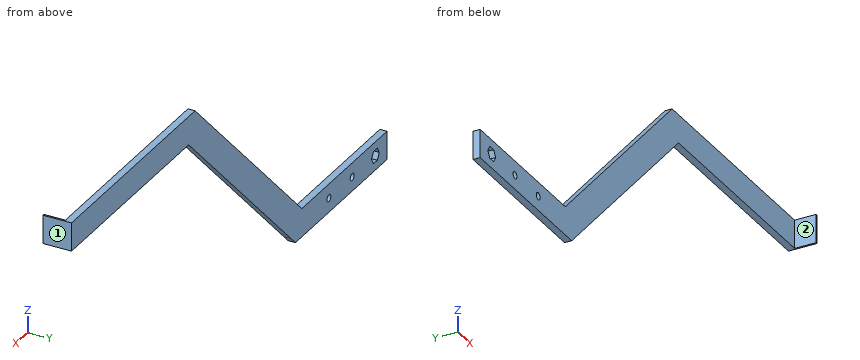
Autodesk Inventor part; units mm, degrees
ref_plane "YZ Plane" through (0, 0, 0) normal (1, 0, 0) x (0, 1, 0)
ref_plane "XZ Plane" through (0, 0, 0) normal (0, 1, 0) x (-1, 0, 0)
ref_plane "XY Plane" through (0, 0, 0) normal (0, 0, 1) x (1, 0, 0)
sketch "Sketch1" plane through (0, 0, 0) normal (0, 1, 0) x (-1, 0, 0)
  line L0 (0, 0) -> (-133.35, 0)
  line L1 (-133.35, 0) -> (-133.35, 25.4)
  line L2 (-133.35, 25.4) -> (0, 25.4)
  line L3 (0, 25.4) -> (0, 0)
  line L4 (-133.35, 25.4) -> (-143.871, 0)
  line L5 (-133.35, 25.4) -> (-105.8572, 25.4) construction
  line L6 (-133.35, 25.4) -> (-151.3105, 7.4395)
  line L7 (-133.35, 25.4) -> (-107.95, 25.4) construction
  line L8 (-151.3105, 7.4395) -> (-143.871, 0)
  line L9 (-133.35, 25.4) -> (-151.3105, 7.4395)
  line L10 (-151.3105, 7.4395) -> (-318.9899, 175.1188)
  line L11 (-318.9899, 175.1188) -> (-301.0293, 193.0793)
  line L12 (-301.0293, 193.0793) -> (-133.35, 25.4)
  circle A0 centre (-12.7, 12.7) radius 6.35
  line L13 (-318.9899, 175.1188) -> (-509.4899, 175.1188)
  line L14 (-509.4899, 175.1188) -> (-509.4899, 200.5188)
  line L15 (-509.4899, 200.5188) -> (-318.9899, 200.5188)
  line L16 (-318.9899, 200.5188) -> (-318.9899, 175.1188)
  line L17 (-318.9899, 175.1188) -> (-308.4688, 200.5188)
  line L18 (-308.4688, 200.5188) -> (-318.9899, 200.5188)
  line L19 (-308.4688, 200.5188) -> (-301.0293, 193.0793)
  line L20 (-133.35, 0) -> (-143.871, 0)
  dimension "d0" = 133.35
  dimension "d1" = 25.4
  dimension "d2" = 112.5
  dimension "d3" = 25.4
  dimension "d4" = 135
  dimension "d5" = 237.1344
  dimension "d6" = 12.7
  dimension "d7" = 190.5
  dimension "d8" = 25.4
extrude "Extrusion1" add sketch "Sketch1" along normal blind 6.35
sketch "Sketch2" plane through (509.4899, 0, 200.5188) normal (1, 0, 0) x (0, 0, -1)
  line L0 (0, 6.35) -> (25.4, 6.35)
  line L1 (25.4, 6.35) -> (25.4, -19.05)
  line L2 (25.4, -19.05) -> (0, -19.05)
  line L3 (0, -19.05) -> (0, 6.35)
  point P0 (200.5188, 0)
  dimension "d11" = 25.4
  dimension "d12" = 25.4
extrude "Extrusion2" add sketch "Sketch2" along normal blind 1.5875
sketch "Sketch3" plane through (0, 0, 0) normal (-1, 0, 0) x (0, 0, 1)
  line L0 (0, 0) -> (25.4, 0)
  line L1 (25.4, 0) -> (25.4, 6.35)
  line L2 (0, 6.35) -> (25.4, 6.35)
  line L3 (0, 0) -> (0, 6.35)
extrude "Extrusion3" add sketch "Sketch3" along normal blind 44.45
sketch "Sketch6" plane through (0, 6.35, 0) normal (0, 1, 0) x (1, 0, 0)
  circle A0 centre (12.7, -12.7) radius 6.35
  line L0 (318.9899, -175.1188) -> (511.0774, -175.1188)
  line L1 (12.7, -12.7) -> (12.7, -6.35)
  line L2 (16.3662, -6.35) -> (20.0323, -12.7)
  line L3 (20.0323, -12.7) -> (16.3662, -19.05)
  line L4 (16.3662, -19.05) -> (9.0338, -19.05)
  line L5 (9.0338, -19.05) -> (5.3677, -12.7)
  line L6 (5.3677, -12.7) -> (9.0338, -6.35)
  line L7 (9.0338, -6.35) -> (16.3662, -6.35)
  point P0 (0, 0)
extrude "Extrusion5" cut sketch "Sketch6" against normal blind 6.35 contours A0 L2 L3 | A0 L7 L2 | L3 L4 A0 | A0 L6 L7 | L4 L5 A0 | A0 L5 L6
sketch "Sketch8" plane through (0, 6.35, 0) normal (0, 1, 0) x (1, 0, 0)
  line L0 (143.871, 0) -> (-44.45, 0)
  line L1 (-44.45, -25.4) -> (-44.45, 0)
  line L2 (318.9899, -175.1188) -> (511.0774, -175.1188)
  line L3 (-44.45, -12.7) -> (12.7, -12.7)
  line L4 (12.7, -12.7) -> (12.7, 0)
  line L5 (12.7, -12.7) -> (-25.4, -12.7)
  line L6 (-25.4, -12.7) -> (50.8, -12.7)
  circle A0 centre (-25.4, -12.7) radius 3.175
  circle A1 centre (50.8, -12.7) radius 3.175
  point P0 (0, 0)
  dimension "d29" = 57.15
  dimension "d30" = 38.1
  dimension "d31" = 76.2
  dimension "d32" = 0
  dimension "d33" = 6.35
  dimension "d34" = 6.35
extrude "Extrusion7" cut sketch "Sketch8" against normal blind 25.4 contours A1 | A0 L3 | L3 A0
sketch "Sketch9" plane through (0, 6.35, 0) normal (0, 1, 0) x (1, 0, 0)
  circle A0 centre (50.8, -12.7) radius 3.175
  circle A1 centre (-25.4, -12.7) radius 3.175
  line L0 (-44.45, 0) -> (0, 0)
  line L1 (0, 0) -> (0, -25.4)
  line L2 (0, -25.4) -> (-44.45, -25.4)
  line L3 (-44.45, -25.4) -> (-44.45, 0)
  line L4 (0, -12.7) -> (12.7, -12.7)
  line L5 (12.7, -12.7) -> (50.8, -12.7)
  line L6 (50.8, -12.7) -> (88.9, -12.7)
  line L7 (50.8, -12.7) -> (88.9, -12.7) construction
  circle A2 centre (88.9, -12.7) radius 3.175
  dimension "d37" = 44.45
  dimension "d38" = 25.4
  dimension "d39" = 38.1
  dimension "d40" = 0
  dimension "d41" = 6.35
extrude "Extrusion8" cut sketch "Sketch9" against normal blind 25.4 contours L1 L2 L3 L0 | A2
sketch "Sketch10" plane through (0, 6.35, 0) normal (-1, 0, 0) x (0, 0, 1)
  line L0 (25.4, -6.35) -> (0, -6.35)
  line L1 (25.4, 0) -> (25.4, -6.35)
  line L2 (0, 0) -> (25.4, 0)
  line L3 (0, -6.35) -> (0, 0)
extrude "Extrusion9" add sketch "Sketch10" along normal blind 6.35
sketch "Sketch11" plane through (0, 6.35, 0) normal (0, 1, 0) x (1, 0, 0)
  line L0 (-6.35, -25.4) -> (-6.35, 0)
  line L1 (5.3677, -12.7) -> (9.0338, -6.35)
  line L2 (9.0338, -6.35) -> (16.3662, -6.35)
  line L3 (16.3662, -6.35) -> (20.0323, -12.7)
  line L4 (20.0323, -12.7) -> (16.3662, -19.05)
  line L5 (16.3662, -19.05) -> (9.0338, -19.05)
  line L6 (9.0338, -19.05) -> (5.3677, -12.7)
  line L7 (-6.35, -12.7) -> (12.7, -12.7)
  line L8 (12.7, -12.7) -> (6.35, -12.7)
  line L9 (12.7, -12.7) -> (19.05, -12.7) construction
  line L10 (6.35, -12.7) -> (9.525, -7.2007)
  line L11 (9.525, -7.2007) -> (15.875, -7.2007)
  line L12 (15.875, -7.2007) -> (19.05, -12.7)
  line L13 (19.05, -12.7) -> (15.875, -18.1993)
  line L14 (15.875, -18.1993) -> (9.525, -18.1993)
  line L15 (9.525, -18.1993) -> (6.35, -12.7)
  point P0 (0, 0)
  dimension "d46" = 6.35
  dimension "d47" = 180
extrude "Extrusion10" add sketch "Sketch11" against normal blind 6.35
properties part number "Z-PickupArm-R"
The listing builds one solid part. Answer for the finished solid, in the listing's coordinates (mm). Face numbers are marked on the shaded views. A direction names the side the tool comes from. Give positions to 0.01 mm unless a question says otherwise; leave off trailing zeros. Order: outer loops, then holes, each group sorted by start corner. A loop starts at its lowest first (then second) coordinate and runs counter-clockwise, first axis right, second up. Notation, with made-up numbers: (57, 89.25) -> (81, 89.25) arc R22 ccw to (81, 115.25) -> close; hole circle Ø10 at (-40, 48). An arc over 180 degrees is marked (long way). One line per item, written item: value.
1) Find section A-A, the plane x = 367.5. Determine the outline of the cut face in (y, z).
Reported:
outline: (0, 175.12) -> (6.35, 175.12) -> (6.35, 200.52) -> (0, 200.52) -> close
2) A tool of negligible diameter and unlimited length cuts with its end or side. For the marked faces 1 and 2, from which of +Z, -Z, +X, -X, +Y, -Y can it reach the whole face along a straight path? Write none if from no direction.
Reported:
face 1: +Z, -Z, +X, +Y, -Y
face 2: +Z, -Z, -X, -Y
3) Flat-ended cylindrical pins translate along their axes: P1, Ø9.5, axis at y = -7, z = 189, coming from the -X side; P2, Ø7, axis at x = 12, y = 2.5, coming from the +Z side; P3, Ø7, axis at x = 12.5, y = 4, coming from the -Z side. Find the tip coordinate at first contact, or state that the pin passes through.
Reported:
P1: stops at x = 509.49
P2: stops at z = 25.4
P3: stops at z = 0
4) Find section B-B, the plane y = -12.5. Determine the outline of the cut face in (x, z), plus the area to 3 significant figures.
Reported:
outline: (509.49, 175.12) -> (511.08, 175.12) -> (511.08, 200.52) -> (509.49, 200.52) -> close
area: 40.3 mm^2
5) Find the intervals of material crossed by line 1 (Z direction, x = 88.9, y = 2.5) (3 decimals); line 2 (Z direction, x = 335, y = 1); line 3 (Z direction, x = 73, y = 1.25), in increasing order.
Reported:
line 1: z = 0 to 9.525, 15.875 to 25.4
line 2: z = 175.12 to 200.52
line 3: z = 0 to 25.4
